Design review of the part built by this model. Coordinates are the model's own, in mm. A direction names the side the tool comes from. Give positions to 0.01 mm unless a question says otherwise; leave off trailing zeros. Loops run counter-clockwise (first coordinate to the right, second up) from the corner with the lowest first, then second, coordinate; pieces in that order, holes last. Notation, with made-up numbers: (83.25, -14.75) -> (126.25, -14.75) arc R10 cw to (126.25, -8.75) -> close; hole circle Ø8 at (1.5, -25.75). An arc over 180 degrees is marked (long way). Answer in a Markdown table with one row per item. Add a question column.
(1) Consider section B-B on x = -79. Write out the cut boundary in (y, z).
(2) For faces 3 (the flat face through (18, 0, 5)), 4 (the cylindrical face through (-119.37, -81.74, 1.08)), 5 (the flat face through (18, 3, 0)), list the 3-axis set-ups (+Z, -Z, +X, -X, +Y, -Y) from which the entire face can be reached by the end or side of a thin tool; tool diameter is ignored.
(3) Consider section A-A on y = 27. Write out the cut boundary in (x, z), then the cut area to 3 significant figures.
(4) Draft analysis for pull direction X (two halves, no side actions). For faces 1 (the flat face through (18, -79, 10)), 2 (the flat face through (-117, 82, 2.2)), state which applies: +X half, -X half, draft (parallel to the pull), parting line (faces both ways), or undercut.
(5) For line 1 (X direction, y = -8.5, z = 6.25); line 2 (Y direction, x = 120, z = 8.5); line 3 (X direction, y = 82.5, z = 9.25), list the stretches that pass through material, from the lowest coordinate up.
(6) For pin 1 (2 mm diameter, centred on x = 79.5, y = 43.5, fed in from +Z); pin 2 (1.5 mm diameter, centred on y = -7.5, z = 6.5, fed in from +X); pin 3 (5.5 mm diameter, centred on y = 17, z = 8.5, fed in from -X); pin 4 (2.5 mm diameter, centred on x = -115.27, y = -80.45, fed in from +Z) (3 decimals), all flat-tipped, find the tip position at first contact; note any pin that passes through.
(7) Consider section C-C on z = 8.5. Write out the cut boundary in (x, y).
from build123d import *

# Parameters (mm, degrees)
SKIZZE1_W                                           = 300
SKIZZE1_H                                           = 194.5
AUFSATZ_LINEAR_AUSTRAGEN1_DEPTH                     = 5
SKIZZE2_W                                           = 290
SKIZZE2_H                                           = 184.5
SKIZZE2_W_2                                         = 250
SKIZZE2_H_2                                         = 149.5
AUFSATZ_LINEAR_AUSTRAGEN2_DEPTH                     = 5
STIRNSENKUNG_F_R_M4_SENKSCHRAUBE_KOPF_B_D           = 4.5
STIRNSENKUNG_F_R_M4_SENKSCHRAUBE_KOPF_B_CBORE_D     = 8.6
STIRNSENKUNG_F_R_M4_SENKSCHRAUBE_KOPF_B_CBORE_DEPTH = 2.2
SPIEGELN2_COPY_1_D                                  = 4.5
SPIEGELN2_COPY_1_CBORE_D                            = 8.6
SPIEGELN2_COPY_1_CBORE_DEPTH                        = 2.2


with BuildPart() as part:
    # Skizze1 → Aufsatz-Linear austragen1 (new body)
    with BuildSketch(Plane.XY):
        with Locations((19.733299505, 1.797169811)):
            Rectangle(SKIZZE1_W, SKIZZE1_H)
    extrude(amount=AUFSATZ_LINEAR_AUSTRAGEN1_DEPTH)

    # Skizze2 → Aufsatz-Linear austragen2 (add)
    with BuildSketch(Plane.XY.offset(5)):
        with Locations((19.733299505, 1.797169811)):
            Rectangle(SKIZZE2_W, SKIZZE2_H)
        with Locations((19.733299505, -0.702830189)):
            Rectangle(SKIZZE2_W_2, SKIZZE2_H_2, mode=Mode.SUBTRACT)
    extrude(amount=AUFSATZ_LINEAR_AUSTRAGEN2_DEPTH)

    # Stirnsenkung für M4 Senkschraube (Kopf Button)1 (through all)
    with Locations(Plane(origin=(0, 0, 0), x_dir=(-1, 0, 0), z_dir=(0, 0, -1))):
        with Locations((115.266700495, 84.047169811)):
            stirnsenkung_f_r_m4_senkschraube_kopf_b = CounterBoreHole(STIRNSENKUNG_F_R_M4_SENKSCHRAUBE_KOPF_B_D / 2, STIRNSENKUNG_F_R_M4_SENKSCHRAUBE_KOPF_B_CBORE_D / 2, STIRNSENKUNG_F_R_M4_SENKSCHRAUBE_KOPF_B_CBORE_DEPTH)

    # Spiegeln1: Stirnsenkung für M4 Senkschraube (Kopf Button)1 across plane
    add(stirnsenkung_f_r_m4_senkschraube_kopf_b.mirror(Plane.ZX.offset(1.797169811)), mode=Mode.SUBTRACT)

    # Spiegeln2: Stirnsenkung für M4 Senkschraube (Kopf Button)1 across plane
    add(stirnsenkung_f_r_m4_senkschraube_kopf_b.mirror(Plane(origin=(19.733299505, 0, 0), x_dir=(0, 0, 1), z_dir=(1, 0, 0))), mode=Mode.SUBTRACT)

    # Spiegeln2 copy 1 (through all)
    with Locations(Plane(origin=(39.46659901, 3.594339623, 0), x_dir=(1, 0, 0), z_dir=(0, 0, -1))):
        with Locations((115.266700495, 84.047169811)):
            CounterBoreHole(SPIEGELN2_COPY_1_D / 2, SPIEGELN2_COPY_1_CBORE_D / 2, SPIEGELN2_COPY_1_CBORE_DEPTH)


solid = part.part
Values follow:
| question | item | result |
|---|---|---|
| 1 | outline | (-95.45, 0) -> (99.05, 0) -> (99.05, 5) -> (94.05, 5) -> (94.05, 10) -> (74.05, 10) -> (74.05, 5) -> (-75.45, 5) -> (-75.45, 10) -> (-90.45, 10) -> (-90.45, 5) -> (-95.45, 5) -> close |
| 2 | face 3 | +Z |
| 2 | face 4 | -Z |
| 2 | face 5 | -Z, +X, -X, +Y, -Y |
| 3 | outline | (-130.27, 0) -> (169.73, 0) -> (169.73, 5) -> (164.73, 5) -> (164.73, 10) -> (144.73, 10) -> (144.73, 5) -> (-105.27, 5) -> (-105.27, 10) -> (-125.27, 10) -> (-125.27, 5) -> (-130.27, 5) -> close |
| 3 | area | 1,700 mm2 |
| 4 | face 1 | draft |
| 4 | face 2 | undercut |
| 5 | line 1 | -125.27 to -105.27, 144.73 to 164.73 |
| 5 | line 2 | -90.45 to -75.45, 74.05 to 94.05 |
| 5 | line 3 | -125.27 to -116.9, -113.63 to 153.1, 156.37 to 164.73 |
| 6 | pin 1 | z = 5 |
| 6 | pin 2 | x = 164.73 |
| 6 | pin 3 | x = -125.27 |
| 6 | pin 4 | through |
| 7 | outline | (-125.27, -90.45) -> (164.73, -90.45) -> (164.73, 94.05) -> (-125.27, 94.05) -> close; hole circle Ø4.5 at (-115.27, -80.45); hole circle Ø4.5 at (-115.27, 84.05); hole (-105.27, -75.45) -> (144.73, -75.45) -> (144.73, 74.05) -> (-105.27, 74.05) -> close; hole circle Ø4.5 at (154.73, -80.45); hole circle Ø4.5 at (154.73, 84.05) |
